from build123d import *

# Parameters (mm, degrees)
SKETCH1_R      = 25.273
SKETCH1_R_2    = 14.88313
SKETCH1_R_3    = 1.8415
EXTRUDE1_DEPTH = 9.525
SKETCH2_W      = 5.0939162
SKETCH2_H      = 11.293845459


with BuildPart() as part:
    # Sketch1 → Extrude1 (new body)
    with BuildSketch(Plane(origin=(0, 0, 0), x_dir=(1, 0, 0), z_dir=(0, 1, 0))):
        with Locations(Location((0, 0, 0), (0, 0, 90))):
            Circle(SKETCH1_R)
        with Locations(Location((0, 0, 0), (0, 0, 90))):
            Circle(SKETCH1_R_2, mode=Mode.SUBTRACT)
        with Locations(Location((0, 20.7772, 0), (0, 0, 90))):
            Circle(SKETCH1_R_3, mode=Mode.SUBTRACT)
        with Locations(Location((0, -20.7772, 0), (0, 0, 90))):
            Circle(SKETCH1_R_3, mode=Mode.SUBTRACT)
        with Locations(Location((20.7772, 0, 0), (0, 0, 90))):
            Circle(SKETCH1_R_3, mode=Mode.SUBTRACT)
        with Locations(Location((-20.7772, 0, 0), (0, 0, 90))):
            Circle(SKETCH1_R_3, mode=Mode.SUBTRACT)
    extrude(amount=EXTRUDE1_DEPTH)

    # Sketch2 → Cut-Revolve1 (revolve, cut)
    with BuildSketch(Plane(origin=(0, 0, 0), x_dir=(0, 0, -1), z_dir=(1, 0, 0)), mode=Mode.PRIVATE) as cut_revolve1_sk:
        with Locations((-27.5024581, 7.93292273)):
            Rectangle(SKETCH2_W, SKETCH2_H)
    revolve(cut_revolve1_sk.sketch.rotate(Axis((0, 0, 0), (0, 1, 0)), 180), axis=Axis((0, 0, 0), (0, 1, 0)), mode=Mode.SUBTRACT)


solid = part.part
The listing builds one solid part. Answer for the finished solid, in the listing's coordinates (mm). A direction names the side the tool comes from. Coordinates: 2 decimals unless noted, no trailing zeros. Write each loop counter-clockwise with the first axis right and the second up, starting at its lowest first coordinate (ties: lowest second). Pieces come first, ordered by that corner, then holes. Notation, with made-up numbers: M -29.75,64.25 L -8.75,64.25 A9 ccw -8.75,71.25 Z; hole C -18.75,75.25 d4. An arc over 180 degrees is marked long. Use one line per item in the form item = value.
Item 1: Find section A-A, the plane z = 0. Give the number of separate pieces and of enclosed holes in the cut face, plus the area to 3 significant figures.
Model answer:
separate_pieces = 4
enclosed_holes = 0
area = 123 mm2
Item 2: For faces 1 (the face through (24.36, 5.96, 5.41)), 2 (the face through (-0.081, 4.696, 22.617)), determine the directions among +Z, -Z, +X, -X, +Y, -Y from which every point of the face is accessible in a straight line to the end or side of a thin tool.
Model answer:
face_1 = +Y
face_2 = +Y, -Y
Item 3: The mould has two halves that part along X. Classify faces 3 (the face through (-21.33, 4.696, -1.756)), 4 (the face through (9.68, 1.127, -23.346)), 5 (the face through (11, 9.525, -11)): released by +X, released by -X, zero draft, split by the parting line, or undercut.
Model answer:
face_3 = undercut
face_4 = split by the parting line
face_5 = zero draft
Item 4: Find the intervals of material crossed by probe 1 along X at (y, z) = (3.75, 0); probe 2 along Z at (x, y) = (0.5, 4.25); probe 3 along Z at (x, y) = (1, 9), in increasing order.
Model answer:
probe_1 = -24.96 to -22.62, -18.94 to -14.88, 14.88 to 18.94, 22.62 to 24.96
probe_2 = -24.95 to -22.55, -19 to -14.87, 14.87 to 19, 22.55 to 24.95
probe_3 = -24.94 to -22.32, -19.23 to -14.85, 14.85 to 19.23, 22.32 to 24.94
Item 5: Given P1, Ø4, axis at y = 5.5, z = 1, coming from the -X side; P2, Ø4, axis at x = 19, y = 7.5, coming from the -Z side; P3, Ø2, axis at x = 0, z = -20.78, coming from the +Y side, each flat-ended and moving along its own axis, determine where each tip first touches the part or whether it passes through.
Model answer:
P1 = -24.96
P2 = -18.27
P3 = through
Item 6: Find section D-D, the plane x = -10. Give the vertices of the cut face in (y, z) (3 decimals), plus the area to 3 significant figures.
Model answer:
outline = M 0,-23.21 L 2.286,-23.21 L 2.286,-22.864 L 9.525,-22.864 L 9.525,-11.023 L 0,-11.023 Z; M 0,11.023 L 9.525,11.023 L 9.525,22.864 L 2.286,22.864 L 2.286,23.21 L 0,23.21 Z
area = 227 mm2
